Autodesk Inventor part; units mm, degrees
ref_plane "Work Plane1" through (0, 0, 1.5) normal (0, 0, -1) x (-1, 0, 0)
ref_plane "YZ Plane" through (0, 0, 0) normal (1, 0, 0) x (0, 1, 0)
ref_plane "XZ Plane" through (0, 0, 0) normal (0, 1, 0) x (-1, 0, 0)
sketch "Sketch1" plane through (0, 0, 0) normal (0, 0, 1) x (1, 0, 0)
  circle A0 centre (0, 0) radius 2.35
  dimension "d0" = 4.7
extrude "Extrusion1" add sketch "Sketch1" along normal blind 7
chamfer "Chamfer1" distance 0.6 angle 45 1 edges at (-2.35, 0, 7)
sketch "Sketch2" plane through (0, 0, 0) normal (0, 0, -1) x (-1, 0, 0)
  circle A0 centre (0, 0) radius 1.5
  dimension "d6" = 3
extrude "Extrusion2" cut sketch "Sketch2" against normal through all
sketch "Sketch3" plane through (0, 0, 0) normal (0, 0, -1) x (-1, 0, 0)
  circle A0 centre (0, 0) radius 2.65
  dimension "d11" = 5.3
extrude "Extrusion3" add sketch "Sketch3" against normal blind 0.01
chamfer "Chamfer2" distance 0.3 angle 45 1 edges at (-2.35, 0, 0.01)
sketch "Sketch4" plane through (0, 0, 0.01) normal (0, 0, 1) x (1, 0, 0)
  circle A0 centre (0, 0) radius 1.5
extrude "Extrusion4" cut sketch "Sketch4" against normal through all
ref_plane "Work Plane1" through (0, 0, 1.5) normal (0, 0, -1) x (-1, 0, 0)
sketch "Sketch6" plane through (0, 0, 0) normal (1, 0, 0) x (0, 1, 0)
  line L0 (2.35, 0.31) -> (2.35, 6.4)
  line L1 (3.71, 1.5) -> (-3.71, 1.5)
  circle A0 centre (2.4109, 1.7672) radius 0.5891
  line L2 (2.9359, 1.5) -> (2.35, 1.5)
  line L3 (2.35, 1.5) -> (2.35, 2.3531)
  line L4 (0, -1.4) -> (0, 8.4)
  point P0 (0, 0)
  dimension "d18" = 3
sketch "Sketch5" plane through (0, 0, 1.5) normal (0, 0, -1) x (-1, 0, 0)
  circle A0 centre (0, 0) radius 2.35
  circle A1 centre (0, 0) radius 2.35
sweep "Sweep1" add profiles "Sketch6" path "Sketch5" picked at (2.489, 2.0554) path curves A0 contours L0 A0 L1
properties part number "pop_PSZROX-0315"
Read the model definition and answer for the solid it produces. Units are mm, in the model's axes. Give positions to 0.01 mm unless a question says otherwise; leave off trailing zeros. Write each loop counter-clockwise with the first axis right and the second up, starting at its lowest first coordinate (ties: lowest second). Pieces come first, ordered by that corner, then holes. Notation, with made-up numbers: M 14.25,-21 L 67.25,-21 A20 cw 67.25,5 Z; hole C 88,40.25 d6. An arc over 180 degrees is marked long. Put each result on its own line as item: value. Start each with the question number.
1. For a pull along Z with two mould halves and no side action, classify faces 1 (the cylindrical face through (-0.509, 2.294, 0.897)), 2 (the cylindrical face through (-0.509, 2.294, 4.348)), 3 (the flat face through (0, -2, 0)) as released by +Z, released by -Z, zero draft, split by the parting line, or undercut.
2. Consider line 1 along Y through (x, z) = (0, 5.25); line 2 along Y through (x, z) = (-0.9, 3); line 3 along X through (y, z) = (0, 0.05). Determine where each line is inside the solid, lowest interval first.
3. This flat-tipped pin is pushed along its axis until it touches: pin 1 Ø2.5 at (x, y) = (0, 0) entering from -Z. Where does it stop, or does it pass through?
4. The part is cut by section A-A, the plane z = 3.25. Give the vertices of the cut face in (x, y).
Final values:
1. face 1: undercut
1. face 2: zero draft
1. face 3: released by -Z
2. line 1: y = -2.35 to -1.5, 1.5 to 2.35
2. line 2: y = -2.17 to -1.2, 1.2 to 2.17
2. line 3: x = -2.61 to -1.5, 1.5 to 2.61
3. pin 1: passes through
4. outline: C 0,0 d4.7; hole C 0,0 d3
